Build history of the part. All positions in model axes, mm. A direction names the side the tool comes from. Give positions to 0.01 mm unless a question says otherwise; leave off trailing zeros. Write each loop counter-clockwise with the first axis right and the second up, starting at its lowest first coordinate (ties: lowest second). Pieces come first, ordered by that corner, then holes. Notation, with made-up numbers: (41, 2.5) -> (66, 2.5) arc R27 ccw to (66, 40.5) -> close; hole circle Ø9 at (-36, -31). An arc over 180 degrees is marked (long way). Put each result on its own line as item: value.
from build123d import *

# Parameters (mm, degrees)
SKETCH1_W                = 7
SKETCH1_H                = 5
BOSS_EXTRUDE1_DEPTH      = 5
HOLE1_D                  = 1.05
HOLE1_CBORE_D            = 1.3
HOLE1_CBORE_DEPTH        = 1.2
SKETCH20_W               = 5
SKETCH20_H               = 2.5
CUT_EXTRUDE11_DEPTH      = 2
M1_0X0_25_TAPPED_HOLE1_D = 0.75
SKETCH37_W               = 5
SKETCH37_H               = 2.5
CUT_EXTRUDE13_DEPTH      = 2
CUT_EXTRUDE15_DEPTH      = 3
CUT_EXTRUDE16_DEPTH      = 9.124038405
SKETCH44_W               = 1.020368792
SKETCH44_H               = 0.499253319
CUT_EXTRUDE17_DEPTH      = 10.197034161


with BuildPart() as part:
    # Sketch1 → Boss-Extrude1 (new body)
    with BuildSketch(Plane(origin=(0, 4, 0), x_dir=(-1, 0, 0), z_dir=(0, 1, 0))):
        with Locations((-3.5, 2.5)):
            Rectangle(SKETCH1_W, SKETCH1_H)
    extrude(amount=-BOSS_EXTRUDE1_DEPTH)

    # Hole1 (through all)
    with Locations(Plane(origin=(0, 0, 0), x_dir=(-1, 0, 0), z_dir=(0, 0, -1))):
        with Locations((-5.7, 0.5), (-0.7, 0.5)):
            CounterBoreHole(HOLE1_D / 2, HOLE1_CBORE_D / 2, HOLE1_CBORE_DEPTH)

    # Sketch20 → Cut-Extrude11 (cut)
    with BuildSketch(Plane(origin=(7, 0, 0), x_dir=(0, 0, -1), z_dir=(1, 0, 0))):
        with Locations((-2.5, 2.75)):
            Rectangle(SKETCH20_W, SKETCH20_H)
    extrude(amount=-CUT_EXTRUDE11_DEPTH, mode=Mode.SUBTRACT)

    # M1.0x0.25 Tapped Hole1 (through all)
    with Locations(Plane(origin=(0, 0, 0), x_dir=(-1, 0, 0), z_dir=(0, 0, -1))):
        with Locations((-3.2, 0.5)):
            Hole(M1_0X0_25_TAPPED_HOLE1_D / 2)

    # Sketch37 → Cut-Extrude13 (cut)
    with BuildSketch(Plane.ZY):
        with Locations((2.5, 2.752068207)):
            Rectangle(SKETCH37_W, SKETCH37_H)
    extrude(amount=-CUT_EXTRUDE13_DEPTH, mode=Mode.SUBTRACT)

    # Sketch41 → Cut-Extrude15 (cut)
    with BuildSketch(Plane(origin=(0, 4, 0), x_dir=(1, 0, 0), z_dir=(0, 1, 0))):
        Polygon((5, -2.6), (3.822078101, -2.05), (3.822078101, -4.55), (5, -4), align=None)
    extrude(amount=-CUT_EXTRUDE15_DEPTH, mode=Mode.SUBTRACT)

    # Sketch43 → Cut-Extrude16 (cut, through all)
    with BuildSketch(Plane.ZY.offset(-2)):
        Polygon((0, 2.250519753), (0.574456265, 1.850519753), (0.574456265, 3.650519753), (0, 3.250519753), align=None)
    extrude(amount=-CUT_EXTRUDE16_DEPTH, mode=Mode.SUBTRACT)

    # Sketch44 → Cut-Extrude17 (cut, through all)
    with BuildSketch(Plane(origin=(0, 0, 0.574456265), x_dir=(-1, 0, 0), z_dir=(0, 0, -1))):
        with Locations((-2.510184396, 2.500893094)):
            Rectangle(SKETCH44_W, SKETCH44_H)
    extrude(amount=-CUT_EXTRUDE17_DEPTH, mode=Mode.SUBTRACT)


solid = part.part
1) Pull direction X, two halves, no side cores. Call faces 1 (the flat face through (5, 2.8, 4.5)), 2 (the flat face through (4.4, 2.52, 4.28)), 3 (the flat face through (1, 1.502, 2)): released by +X, released by -X, zero draft, split by the parting line, or undercut.
Filled sheet:
face 1: released by +X
face 2: undercut
face 3: zero draft
2) Slice it at A-A (y = 0.5). Write the cut outline in (x, z) (3 decimals), plus the area to 4 significant figures.
Filled sheet:
outline: (0, 0) -> (0.05, 0) -> (0.05, 1.2) -> (0.175, 1.2) -> (0.175, 5) -> (0, 5) -> close; (1.225, 1.2) -> (1.35, 1.2) -> (1.35, 0) -> (2.825, 0) -> (2.825, 5) -> (1.225, 5) -> close; (3.575, 0) -> (5.05, 0) -> (5.05, 1.2) -> (5.175, 1.2) -> (5.175, 5) -> (3.575, 5) -> close; (6.225, 1.2) -> (6.35, 1.2) -> (6.35, 0) -> (7, 0) -> (7, 5) -> (6.225, 5) -> close
area: 20.15 mm2
3) Tool access for faces 4 (the flat face through (2.5, 2.751, 2.8)), 5 (the flat face through (5, 3, 1)), 6 (the flat face through (3.822, 3, 3)), 7 (the flat face through (2, 3, 2)), 8 (the cylindrical face through (5.1, 0.25, 0.59)): list every direction of +Z, -Z, +X, -X, +Y, -Y with a clear straight run to the whole face (end or side of a thin tool).
Filled sheet:
face 4: +Z, -Z, -X
face 5: +Z, -Z, +X, +Y
face 6: +Y
face 7: +Z, -Z, -X, +Y
face 8: -Z
4) Wall check: L1, parallel to Y at x = 5.7, z = 0.75; L2, parallel to Y at x = 3.2, z = 2.6 (3 decimals); L3, parallel to Y at x = 1.5, z = 3.4. Give the ranges that are in metal, low to high.
Filled sheet:
L1: -1 to -0.15, 1.15 to 1.5
L2: -1 to 0.125, 0.875 to 4
L3: -1 to 1.5
5) Slice it at D-D (z = 0.45). Write the cut outline in (x, y) (3 decimals), plus the area to 3 significant figures.
Filled sheet:
outline: (0, -1) -> (7, -1) -> (7, 1.5) -> (5, 1.5) -> (5, 1.937) -> (2, 1.937) -> (2, 1.502) -> (0, 1.502) -> close; (2, 3.564) -> (5, 3.564) -> (5, 4) -> (2, 4) -> close; hole circle Ø1.3 at (0.7, 0.5); hole circle Ø0.75 at (3.2, 0.5); hole circle Ø1.3 at (5.7, 0.5)
area: 17.0 mm2
6) Pin check, flat tips, straight feed: pin 1 (1.4 mm diameter, centred on x = 5.7, y = 0.5, fed in from +Z); pin 2 (1.1 mm diameter, centred on y = 2.5, z = 4.5, fed in from +X); pin 3 (1 mm diameter, centred on y = 2.5, z = 3.5, fed in from -X); pin 4 (2 mm diameter, centred on x = 0.5, z = 2.5, fed in from +Y). Stop position of each tip, or through.
Filled sheet:
pin 1: z = 5
pin 2: x = 5
pin 3: x = 2
pin 4: y = 1.5
7) Slice it at C-C (x = 0.7). Write the cut outline in (y, z) (3 decimals).
Filled sheet:
outline: (-1, 0) -> (-0.15, 0) -> (-0.15, 1.2) -> (-0.025, 1.2) -> (-0.025, 5) -> (-1, 5) -> close; (1.025, 1.2) -> (1.15, 1.2) -> (1.15, 0) -> (1.502, 0) -> (1.502, 5) -> (1.025, 5) -> close
8) Slice it at B-B (z = 1.05). Write the cut outline in (x, y) (3 decimals).
Filled sheet:
outline: (0, -1) -> (7, -1) -> (7, 1.5) -> (5, 1.5) -> (5, 4) -> (2, 4) -> (2, 2.751) -> (3.02, 2.751) -> (3.02, 2.251) -> (2, 2.251) -> (2, 1.502) -> (0, 1.502) -> close; hole circle Ø1.3 at (0.7, 0.5); hole circle Ø0.75 at (3.2, 0.5); hole circle Ø1.3 at (5.7, 0.5)
